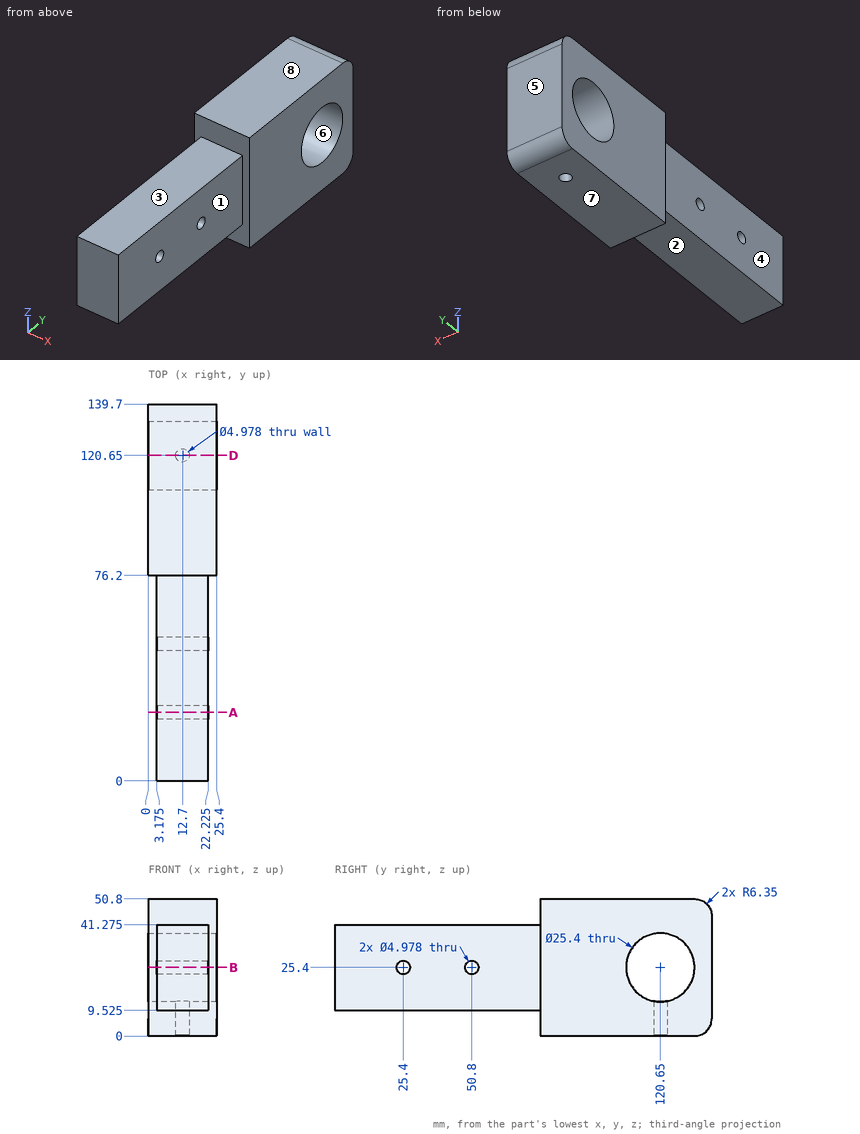
Print and shaded views of the part. All mm, measured from the part's lowest x, y and z. A direction names the side the tool comes from. Coordinates: 2 decimals unless noted, no trailing zeros. Loops run counter-clockwise (first coordinate to the right, second up) from the corner with the lowest first, then second, coordinate; pieces in that order, holes last. Notation, with made-up numbers: M 27.25,-40 L 76.25,-40 A28 ccw 76.25,-10 Z; hole C 33,-37 d7. An arc over 180 degrees is marked long. Use a Markdown table: item, result. Add a question column.
Q1. Pin check, flat tips, straight feed: P1, Ø2, axis at y = 50.5, z = 38, coming from the -X side (3 decimals); P2, Ø4.5, axis at x = 12.7, y = 120.65, coming from the -Z side; P3, Ø8, axis at x = 5, y = 71, coming from the -Z side (3 decimals). Stop position of each tip, or through.
Q2. Which spindle directions (+Z, -Z, +X, -X, +Y, -Y) get a long thin tool onto all of the face, cutting with end or side? Do the marked faces 1, 2, 3 and 4. Say none if no direction does.
Q3. Cut at A-A (y = 25.4). Write the cut outline in (x, z) (1 decimal), and give its area (3 significant figures).
Q4. Mould opens along Z. For the marked faces 5, 6, 7 and 8 say: +Z half, -Z half, draft (parallel to the pull), parting line (faces both ways), or undercut.
Q5. Cut at B-B (z = 25.4). Give the number of separate pieces and of enclosed holes in the cut face, and give its area (3 significant figures).
Q6. Cut at D-D (y = 120.65). Write the cut outline in (x, z), and give its area (3 significant figures).
Q7. Probe L1, parallel to Y at x = 8.25, z = 25.4; L2, parallel to Y at x = 12.7, z = 10.25; L3, parallel to X at y = 40, z = 32.5 (1 decimal). List the from-to ranges inside material, lowest first.
Worked out:
| question | item | result |
|---|---|---|
| 1 | P1 | stops at x = 3.175 |
| 1 | P2 | stops at z = 37.9 |
| 1 | P3 | stops at z = 9.525 |
| 2 | face 1 | +Z, -Z, +X, -Y |
| 2 | face 2 | -Z, +X, -X, -Y |
| 2 | face 3 | +Z, +X, -X, -Y |
| 2 | face 4 | +Z, -Z, -X, -Y |
| 3 | outline | M 3.2,9.5 L 22.2,9.5 L 22.2,22.9 L 3.2,22.9 Z; M 3.2,27.9 L 22.2,27.9 L 22.2,41.3 L 3.2,41.3 Z |
| 3 | area | 510 mm2 |
| 4 | face 5 | draft |
| 4 | face 6 | undercut |
| 4 | face 7 | -Z half |
| 4 | face 8 | +Z half |
| 5 | separate pieces | 4 |
| 5 | enclosed holes | 0 |
| 5 | area | 2,230 mm2 |
| 6 | outline | M 0,0 L 10.21,0 L 10.21,12.7 L 0,12.7 Z; M 0,38.1 L 25.4,38.1 L 25.4,50.8 L 0,50.8 Z; M 15.19,0 L 25.4,0 L 25.4,12.7 L 15.19,12.7 Z |
| 6 | area | 582 mm2 |
| 7 | L1 | y = 0 to 22.91, 27.89 to 48.31, 53.29 to 107.95, 133.35 to 139.7 |
| 7 | L2 | y = 0 to 118.16, 123.14 to 139.7 |
| 7 | L3 | x = 3.2 to 22.2 |
